Source: CAD feature listing. Evaluate the final solid. Frame: model axes, mm. A direction names the side the tool comes from. Round coordinates to 2 decimals unless told otherwise and drop trailing zeros. Loops run counter-clockwise (first coordinate to the right, second up) from the corner with the lowest first, then second, coordinate; pieces in that order, holes last. Notation, with made-up numbers: M 45,-17.5 L 74,-17.5 A31 ccw 74,6.5 Z; hole C -25.75,73.25 d3. An arc over 180 degrees is marked long. Write each question's results on one line, items separated by ' | '. Start each with the question number.
1. Ray query, line 1 (X direction, y = 30.5, z = 0.9); line 2 (Z direction, x = -2, y = -1); line 3 (X direction, y = 3, z = 0.2). Return the intervals inside material, ascending.
2. Section B-B on z = 5.3. Output: boundary loops of the cut face in (x, y).
3. Contact query for flat-ended pins moving along their axis: pin 1 Ø3 at (x, z) = (15, 3.5) entering from +Y; pin 2 Ø1 at (y, z) = (-18, 2.5) entering from +X; pin 3 Ø3 at (y, z) = (-2, 3) entering from -X (3 decimals); pin 4 Ø6 at (x, y) = (0.5, 2) entering from -Z. Output: stop coordinate, or through.
4. Section A-A on x = 0. Output: boundary loops of the cut face in (y, z), and give its area (3 significant figures).
5. Draft query along X for faces 4 (the flat face through (8, 36, 3)), 5 (the flat face through (25, 18, 3)), 6 (the flat face through (17, 33, 3)). Return one class per face: released by +X, released by -X, zero draft, split by the parting line, or undercut.
6. Section D-D on x = -8.5. Output: boundary loops of the cut face in (y, z), and give its area (3 significant figures).
7. Set-up query: faces 1 (the flat face through (-2.26, 8.25, 0.99)), 2 (the flat face through (-17, 33, 3)), 3 (the flat face through (21, 36, 3)). Return all of +Z, -Z, +X, -X, +Y, -Y with unobstructed straight access to the full face (end or side cutting, diameter ignored); none if empty.
8. Section C-C on y = -8. Output: boundary loops of the cut face in (x, z), and give its area (3 significant figures).
from build123d import *

# Parameters (mm, degrees)
SKETCH2_R                = 25
BOSS_EXTRUDE1_DEPTH      = 6
BOSS_EXTRUDE2_START      = -4
BOSS_EXTRUDE2_DEPTH      = 4
BOSS_EXTRUDE4_DEPTH      = 6
SKETCH5_W                = 8
SKETCH5_H                = 6
SKETCH5_W_2              = 6
BOSS_EXTRUDE5_DEPTH      = 6
MOVE_START               = 31
MOVE_FACE1_OUTLINE_W     = 8
MOVE_FACE1_OUTLINE_H     = 6
MOVE_FACE1_OUTLINE_W_2   = 6
MOVE_FACE1_DEPTH         = 5
MOVE_START_2             = 25
MOVE_FACE1_2_OUTLINE_W   = 6
MOVE_FACE1_2_OUTLINE_H   = 6
MOVE_FACE1_2_OUTLINE_W_2 = 10
MOVE_FACE1_2_DEPTH       = 5


# Read off the part's stored shape, not the designer's step: Move Face1
with BuildPart() as part:
    # Sketch2 → Boss-Extrude1 (new body)
    with BuildSketch(Plane.XY):
        Circle(SKETCH2_R)
        with BuildLine():
            Line((-2.73463726, -2.341315668), (-1.8, -14))
            ThreePointArc((-1.8, -14), (0, -15.8), (1.8, -14))
            Line((1.8, -14), (2.73463726, -2.341315668))
            ThreePointArc((2.73463726, -2.341315668), (3.6, 0), (2.73463726, 2.341315668))
            Line((2.73463726, 2.341315668), (1.8, 14))
            ThreePointArc((1.8, 14), (0, 15.8), (-1.8, 14))
            Line((-1.8, 14), (-2.73463726, 2.341315668))
            ThreePointArc((-2.73463726, 2.341315668), (-3.6, 0), (-2.73463726, -2.341315668))
        make_face(mode=Mode.SUBTRACT)
    extrude(amount=BOSS_EXTRUDE1_DEPTH)

    # Sketch3 → Boss-Extrude2 (add)
    with BuildSketch(Plane.XY.offset(6).offset(BOSS_EXTRUDE2_START)):
        with BuildLine():
            Line((2.73463726, 2.341315668), (1.8, 14))
            ThreePointArc((1.8, 14), (0, 15.8), (-1.8, 14))
            Line((-1.8, 14), (-2.73463726, 2.341315668))
            ThreePointArc((-2.73463726, 2.341315668), (-3.6, 0), (-2.73463726, -2.341315668))
            Line((-2.73463726, -2.341315668), (-1.8, -14))
            ThreePointArc((-1.8, -14), (0, -15.8), (1.8, -14))
            Line((1.8, -14), (2.73463726, -2.341315668))
            ThreePointArc((2.73463726, -2.341315668), (3.6, 0), (2.73463726, 2.341315668))
        make_face()
    extrude(amount=BOSS_EXTRUDE2_DEPTH)


with BuildPart() as body_2:
    # Sketch4 → Boss-Extrude4 (new body)
    with BuildSketch(Plane(origin=(0, 0, 0), x_dir=(-1, 0, 0), z_dir=(0, 0, -1))):
        with BuildLine():
            Line((25, 0), (25, 25))
            Line((25, 25), (0, 25))
            ThreePointArc((0, 25), (17.67766953, 17.67766953), (25, 0))
        make_face()
    extrude(amount=-BOSS_EXTRUDE4_DEPTH)


with BuildPart() as body_3:
    # Mirror1: mirrored copy
    add(body_2.part.mirror(Plane.ZY))


with BuildPart() as part_1:
    add(part.part)

    # Combine1: union body 2, body 3
    add(body_2.part)
    add(body_3.part)

    # Sketch5 → Boss-Extrude5 (add)
    with BuildSketch(Plane(origin=(0, 25, 0), x_dir=(1, 0, 0), z_dir=(0, 1, 0))):
        with Locations((21, -3)):
            Rectangle(SKETCH5_W, SKETCH5_H)
        with Locations((-8, -3)):
            Rectangle(SKETCH5_W_2, SKETCH5_H)
        with Locations((8, -3)):
            Rectangle(SKETCH5_W_2, SKETCH5_H)
        with Locations((-21, -3)):
            Rectangle(SKETCH5_W, SKETCH5_H)
    extrude(amount=BOSS_EXTRUDE5_DEPTH)

    # Move Face1 outline → Move Face1 (add)
    with BuildSketch(Plane(origin=(0, 0, 0), x_dir=(1, 0, 0), z_dir=(0, 1, 0)).offset(MOVE_START)):
        with Locations((-21, -3)):
            Rectangle(MOVE_FACE1_OUTLINE_W, MOVE_FACE1_OUTLINE_H)
        with Locations((-8, -3)):
            Rectangle(MOVE_FACE1_OUTLINE_W_2, MOVE_FACE1_OUTLINE_H)
        with Locations((8, -3)):
            Rectangle(MOVE_FACE1_OUTLINE_W_2, MOVE_FACE1_OUTLINE_H)
        with Locations((21, -3)):
            Rectangle(MOVE_FACE1_OUTLINE_W, MOVE_FACE1_OUTLINE_H)
    extrude(amount=MOVE_FACE1_DEPTH)

    # Move Face1 2 outline → Move Face1 2 (add)
    with BuildSketch(Plane(origin=(0, 0, 0), x_dir=(1, 0, 0), z_dir=(0, 1, 0)).offset(MOVE_START_2)):
        with Locations((-14, -3)):
            Rectangle(MOVE_FACE1_2_OUTLINE_W, MOVE_FACE1_2_OUTLINE_H)
        with Locations((0, -3)):
            Rectangle(MOVE_FACE1_2_OUTLINE_W_2, MOVE_FACE1_2_OUTLINE_H)
        with Locations((14, -3)):
            Rectangle(MOVE_FACE1_2_OUTLINE_W, MOVE_FACE1_2_OUTLINE_H)
    extrude(amount=MOVE_FACE1_2_DEPTH)


solid = part_1.part
Taken from the geometry:
1) line 1: -25 to -17, -11 to -5, 5 to 11, 17 to 25 | line 2: 2 to 6 | line 3: -25 to -2.68, 2.68 to 25
2) outline: M -25,0 A25 ccw 25,0 L 25,36 L 17,36 L 17,30 L 11,30 L 11,36 L 5,36 L 5,30 L -5,30 L -5,36 L -11,36 L -11,30 L -17,30 L -17,36 L -25,36 Z
3) pin 1: y = 30 | pin 2: x = 17.85 | pin 3: x = -24.995 | pin 4: z = 0
4) outline: M -25,0 L -15.8,0 L -15.8,2 L 15.8,2 L 15.8,0 L 30,0 L 30,6 L -25,6 Z | area: 267 mm^2
5) face 4: zero draft | face 5: released by +X | face 6: undercut
6) outline: M -23.51,0 L 36,0 L 36,6 L -23.51,6 Z | area: 357 mm^2
7) face 1: -Z | face 2: +Z, -Z, +Y | face 3: +Z, -Z, +X, -X, +Y
8) outline: M -23.69,0 L -2.28,0 L -2.28,2 L 2.28,2 L 2.28,0 L 23.69,0 L 23.69,6 L -23.69,6 Z | area: 275 mm^2
